from build123d import *
from OCP.BRepFilletAPI import BRepFilletAPI_MakeChamfer

# Parameters (mm, degrees)
BOSS_EXTRUDE1_DEPTH      = 0.85
SKETCH3_R                = 0.3
SKETCH3_R_2              = 0.2
SKETCH3_R_3              = 0.225
BOSS_EXTRUDE2_DEPTH      = 0.2
FILLET1_R                = 0.4
CHAMFER1_SIZE            = 1.2
CHAMFER1_SIZE2           = 0.3
FILLET2_R                = 0.4
BOSS_EXTRUDE4_DEPTH      = 0.2
BOSS_EXTRUDE4_DEPTH_BACK = 1.4
SKETCH7_R                = 0.4
BOSS_EXTRUDE5_DEPTH      = 0.2
BOSS_EXTRUDE5_DEPTH_BACK = 1.4
SKETCH8_R                = 0.4
SKETCH6_W                = 0.5
SKETCH6_H                = 1.7
CUT_EXTRUDE1_DEPTH       = 11.924284874
BOSS_EXTRUDE8_DEPTH      = 0.2
BOSS_EXTRUDE8_DEPTH_BACK = 0.6
SKETCH11_W               = 5.1
SKETCH11_H               = 1
BOSS_EXTRUDE9_DEPTH      = 4.85
CUT_EXTRUDE2_DEPTH       = 9.7
BOSS_EXTRUDE11_START     = 0.7
SKETCH16_R               = 0.25
SKETCH16_R_2             = 0.2
BOSS_EXTRUDE11_DEPTH     = 0.4
BOSS_EXTRUDE12_START     = 1.1
SKETCH17_R               = 0.2
SKETCH17_R_2             = 0.25
BOSS_EXTRUDE12_DEPTH     = 0.4
CUT_EXTRUDE3_DEPTH       = 0.4
CUT_EXTRUDE3_DEPTH_BACK  = 1
SKETCH18_W               = 6.7
SKETCH18_H               = 1
BOSS_EXTRUDE13_DEPTH     = 0.1
SCALE1_SCALE             = 2


with BuildPart() as part:
    # Sketch1 → Boss-Extrude1 (new, symmetric)
    with BuildSketch(Plane(origin=(0, 0, 0), x_dir=(1, 0, 0), z_dir=(0, 1, 0))):
        Polygon((-3.35, 0), (-3.35, 10.1), (3.35, 10.1), (3.35, 0), (3.6, 0), (3.6, -2.4), (2.3, -2.4), (2.3, 0), (2.55, 0), (2.55, 8.9), (-2.55, 8.9), (-2.55, 0), (-2.3, 0), (-2.3, -2.4), (-3.6, -2.4), (-3.6, 0), align=None)
    extrude(amount=BOSS_EXTRUDE1_DEPTH, both=True)

    # Sketch3 → Boss-Extrude2 (add, symmetric)
    with BuildSketch(Plane(origin=(0, 0, 0), x_dir=(1, 0, 0), z_dir=(0, 1, 0))):
        Polygon((-2.55, 3.95), (-2.55, 0), (-1.05, 3.95), (1.05, 3.95), (2.55, 0), (2.55, 3.95), (2.55, 4.95), (2.55, 8.9), (1.05, 4.95), (-1.05, 4.95), (-2.55, 8.9), (-2.55, 4.95), align=None)
        with Locations(Location((-2.2, 3.5, 0), (0, 0, 270))):
            Circle(SKETCH3_R, mode=Mode.SUBTRACT)
        with Locations(Location((2.2, 3.5, 0), (0, 0, 90))):
            Circle(SKETCH3_R, mode=Mode.SUBTRACT)
        with Locations(Location((-2.31, 2.4, 0), (0, 0, 270))):
            Circle(SKETCH3_R_2, mode=Mode.SUBTRACT)
        with Locations(Location((-2.31, 6.5, 0), (0, 0, 270))):
            Circle(SKETCH3_R_3, mode=Mode.SUBTRACT)
        with Locations(Location((2.2, 5.4, 0), (0, 0, 270))):
            Circle(SKETCH3_R, mode=Mode.SUBTRACT)
        with Locations(Location((-2.2, 5.4, 0), (0, 0, 90))):
            Circle(SKETCH3_R, mode=Mode.SUBTRACT)
        with Locations(Location((2.31, 2.4, 0), (0, 0, 90))):
            Circle(SKETCH3_R_2, mode=Mode.SUBTRACT)
        with Locations(Location((2.31, 6.5, 0), (0, 0, 90))):
            Circle(SKETCH3_R_3, mode=Mode.SUBTRACT)
    extrude(amount=BOSS_EXTRUDE2_DEPTH, both=True)

    # Fillet1
    fillet1_edges = [part.edges().sort_by_distance(p)[0] for p in [
        (2.95, -0.85, 2.4),
        (-2.95, -0.85, 2.4),
    ]]
    fillet(fillet1_edges, radius=FILLET1_R)

    # Chamfer1: one chamfer whose edges measure the first distance from different faces: ONE call of the kernel's chamfer builder (chamfer() names one face for all edges)
    chamfer1_edges_1 = [part.edges().sort_by_distance(p)[0] for p in [
        (-2.95, 0.85, 2.4),
    ]]
    chamfer1_side_1 = [part.faces().sort_by_distance(p)[0] for p in [
        (-2.95, 0.2, 2.4),
    ]]
    chamfer1_edges_2 = [part.edges().sort_by_distance(p)[0] for p in [
        (2.95, 0.85, 2.4),
    ]]
    chamfer1_side_2 = [part.faces().sort_by_distance(p)[0] for p in [
        (2.95, 0.2, 2.4),
    ]]
    chamfer1 = BRepFilletAPI_MakeChamfer(part.part.solid().wrapped)
    for e in chamfer1_edges_1:
        chamfer1.Add(CHAMFER1_SIZE, CHAMFER1_SIZE2, e.wrapped, chamfer1_side_1[0].wrapped)  # the first distance lies on this face
    for e in chamfer1_edges_2:
        chamfer1.Add(CHAMFER1_SIZE, CHAMFER1_SIZE2, e.wrapped, chamfer1_side_2[0].wrapped)  # the first distance lies on this face
    add(Compound.cast(chamfer1.Shape()), mode=Mode.REPLACE)

    # Fillet2
    fillet2_edges = [part.edges().sort_by_distance(p)[0] for p in [
        (-2.95, 0.85, 2.1),
        (2.95, 0.85, 2.1),
    ]]
    fillet(fillet2_edges, radius=FILLET2_R)

    # Sketch7 → Boss-Extrude4 (add, two sides: drawn at the far end of the back side and taken through both)
    with BuildSketch(Plane.ZY.offset(3.6).offset(-BOSS_EXTRUDE4_DEPTH_BACK)):
        with Locations((1.9, -0.35)):
            Circle(SKETCH7_R)
    extrude(amount=BOSS_EXTRUDE4_DEPTH + BOSS_EXTRUDE4_DEPTH_BACK)

    # Sketch8 → Boss-Extrude5 (add, two sides: drawn at the far end of the back side and taken through both)
    with BuildSketch(Plane(origin=(3.6, 0, 0), x_dir=(0, 0, -1), z_dir=(1, 0, 0)).offset(-BOSS_EXTRUDE5_DEPTH_BACK)):
        with Locations(Location((-1.9, -0.35, 0), (0, 0, 180))):
            Circle(SKETCH8_R)
    extrude(amount=BOSS_EXTRUDE5_DEPTH + BOSS_EXTRUDE5_DEPTH_BACK)

    # Sketch6 → Cut-Extrude1 (cut, through all)
    with BuildSketch(Plane(origin=(0, 0.85, 0), x_dir=(1, 0, 0), z_dir=(0, 1, 0))):
        with Locations((-2.95, -1.55)):
            Rectangle(SKETCH6_W, SKETCH6_H)
        with Locations((2.95, -1.55)):
            Rectangle(SKETCH6_W, SKETCH6_H)
    extrude(amount=-CUT_EXTRUDE1_DEPTH, mode=Mode.SUBTRACT)

    # Sketch11 → Boss-Extrude8 (add, two sides: drawn at the far end of the back side and taken through both)
    with BuildSketch(Plane(origin=(0, 0.2, 0), x_dir=(1, 0, 0), z_dir=(0, 1, 0)).offset(-BOSS_EXTRUDE8_DEPTH_BACK)):
        with Locations((0, 4.45)):
            Rectangle(SKETCH11_W, SKETCH11_H)
    extrude(amount=BOSS_EXTRUDE8_DEPTH + BOSS_EXTRUDE8_DEPTH_BACK)

    # Sketch12 → Boss-Extrude9 (add, symmetric)
    with BuildSketch(Plane(origin=(0, 0, 0), x_dir=(0, 0, -1), z_dir=(1, 0, 0))):
        Polygon((9.124920058, 0.542558475), (10.157357644, -0.931915204), (10.64884887, -0.587769343), (9.960557147, 0.395213111), (12.745674097, 2.345372994), (12.401528235, 2.836864221), align=None)
    extrude(amount=BOSS_EXTRUDE9_DEPTH, both=True)

    # Sketch13 → Cut-Extrude2 (cut)
    with BuildSketch(Plane(origin=(3.35, 0, 0), x_dir=(0, 0, -1), z_dir=(1, 0, 0))):
        Polygon((9.960557147, 0.395213111), (10.1, 0.196068077), (10.1, 0.492852048), align=None)
    extrude(amount=-CUT_EXTRUDE2_DEPTH, mode=Mode.SUBTRACT)

    # Sketch16 → Boss-Extrude11 (add)
    with BuildSketch(Plane.ZY.offset(BOSS_EXTRUDE11_START)):
        Polygon((-9.960557147, 0.395213111), (-12.172267666, 1.943869489), (-10.64884887, -0.587769343), align=None)
        with Locations((-10.322666552, 0.331363452)):
            Circle(SKETCH16_R, mode=Mode.SUBTRACT)
        with Locations((-10.949309365, 0.831182204)):
            Circle(SKETCH16_R_2, mode=Mode.SUBTRACT)
    extrude(amount=BOSS_EXTRUDE11_DEPTH)

    # Sketch17 → Boss-Extrude12 (add)
    with BuildSketch(Plane(origin=(0, 0, 0), x_dir=(0, 0, -1), z_dir=(1, 0, 0)).offset(BOSS_EXTRUDE12_START)):
        Polygon((12.172267666, 1.943869489), (9.960557147, 0.395213111), (10.64884887, -0.587769343), align=None)
        with Locations(Location((10.949309365, 0.831182204, 0), (0, 0, 180))):
            Circle(SKETCH17_R, mode=Mode.SUBTRACT)
        with Locations(Location((10.322666552, 0.331363452, 0), (0, 0, 180))):
            Circle(SKETCH17_R_2, mode=Mode.SUBTRACT)
    extrude(amount=-BOSS_EXTRUDE12_DEPTH)

    # Sketch14 → Cut-Extrude3 (cut, two sides: drawn at the far end of the back side and taken through both)
    with BuildSketch(Plane(origin=(0, -4.414739047, -3.09123356), x_dir=(-1, 0, 0), z_dir=(0, -0.8191520442889928, -0.5735764363510448)).offset(-CUT_EXTRUDE3_DEPTH_BACK)):
        with BuildLine():
            Line((-4.85, 10.696327944), (-2.75, 11.585895676))
            ThreePointArc((-2.75, 11.585895676), (-1.419001054, 10.971909117), (-0.2, 11.785895676))
            Line((-0.2, 11.785895676), (0.2, 11.785895676))
            ThreePointArc((0.2, 11.785895676), (1.419001054, 10.971909117), (2.75, 11.585895676))
            Line((2.75, 11.585895676), (4.85, 10.696327944))
            Line((4.85, 10.696327944), (4.85, 12.785895676))
            Line((4.85, 12.785895676), (-4.85, 12.785895676))
            Line((-4.85, 12.785895676), (-4.85, 10.696327944))
        make_face()
    extrude(amount=CUT_EXTRUDE3_DEPTH + CUT_EXTRUDE3_DEPTH_BACK, mode=Mode.SUBTRACT)

    # Sketch18 → Boss-Extrude13 (add)
    with BuildSketch(Plane(origin=(0, 0.85, 0), x_dir=(1, 0, 0), z_dir=(0, 1, 0))):
        with Locations((0, 9.4)):
            Rectangle(SKETCH18_W, SKETCH18_H)
    extrude(amount=BOSS_EXTRUDE13_DEPTH)


with BuildPart() as part_1:
    # Scale1: scaled about (0, 0, 0)
    add(part.part.scale(SCALE1_SCALE))


solid = part_1.part
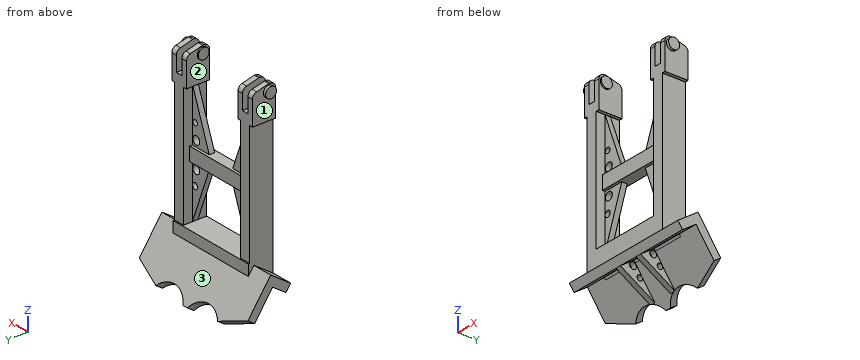
The listing builds one solid part. Answer for the finished solid, in the listing's coordinates (mm). Face numbers are marked on the shaded views. Coordinates: 2 decimals unless noted, no trailing zeros. Write each loop counter-clockwise with the first axis right and the second up, starting at its lowest first coordinate (ties: lowest second). Pieces come first, ordered by that corner, then holes. Notation, with made-up numbers: M 88.5,-1 L 125.5,-1 A23 cw 125.5,12 Z; hole C 33,23 d9. An arc over 180 degrees is marked long. Put each result on its own line as item: value. Start each with the question number.
1. A cutting plane is placed at B-B on x = 3.5. Write down the section's boundary in (y, z).
2. A cutting plane is placed at A-A on z = -13. Count the separate pieces of the cut face and the enclosed holes in it, then the cut area to 3 significant figures.
3. Flat-ended cylindrical pins translate along their axes: P1, Ø1, axis at y = 0.5, z = 2.5, coming from the -X side; P2, Ø2, axis at x = -5.5, z = -7, coming from the +Y side; P3, Ø1, axis at y = 1, z = -11, coming from the +X side. Find the tip coordinate at first contact, or state that the pin passes through.
4. A cutting plane is placed at C-C on z = -17.5. Write down the section's boundary in (x, y).
5. Consider line 1 (X direction, y = 1, z = 1); line 2 (X direction, y = -0.75, z = -1.5); line 3 (Y direction, x = -5.75, z = 1). Determine where each line is inside the solid, lowest interval first. Write a range as from..to.
6. For a pull along X with two mould halves and no side action, classify the marked faces 1, 2 and 3 as pulls with the +X half, pulls with the -X half, needs draft (parallel to the pull), parting line crosses it, or undercut.
Resolved:
1. outline: M -1.86,-20.31 L -1.18,-21.3 L 0.79,-19.92 L 3.77,-24.18 L 4.75,-23.49 L 1.9,-19.41 L 1.9,-17.8 L -1.7,-17.8 L -1.7,-20.2 Z; M -0.8,-9.9 L -0.4,-9.9 L -0.4,-13.59 L 0.4,-13.59 L 0.4,-9.9 L 0.8,-9.9 L 0.8,-7.9 L 0.4,-7.9 L 0.4,-4.21 L -0.4,-4.21 L -0.4,-7.9 L -0.8,-7.9 Z
2. separate pieces: 4
2. enclosed holes: 0
2. area: 12.4 mm2
3. P1: stops at x = -7.2
3. P2: stops at y = 1.7
3. P3: stops at x = 6.7
4. outline: M -6.7,-1.7 L -5.1,-1.7 L -5.1,-0.4 L -4.99,-0.4 L -4.99,0.4 L -5.1,0.4 L -5.1,1.7 L -6.7,1.7 Z; M 4.99,-0.4 L 5.1,-0.4 L 5.1,-1.7 L 6.7,-1.7 L 6.7,1.7 L 5.1,1.7 L 5.1,0.4 L 4.99,0.4 Z
5. line 1: x = -7.2..-4.6, 4.6..7.2
5. line 2: x = -6.7..-5.1, 5.1..6.7
5. line 3: y = -1.7..1.7
6. face 1: pulls with the -X half
6. face 2: undercut
6. face 3: needs draft
